Check sheet for the modelled part. Datum: model origin and axes. Units: mm. A direction names the side the tool comes from. Round coordinates to 2 decimals unless told otherwise and drop trailing zeros. Order: outer loops, then holes, each group sorted by start corner. A loop starts at its lowest first (then second) coordinate and runs counter-clockwise, first axis right, second up.
```python
from build123d import *

# Parameters (mm, degrees)
BOSS_EXTRUDE1_DEPTH         = 2
SKETCH5_R                   = 4
SKETCH5_R_2                 = 1.998542518
BOSS_EXTRUDE2_DEPTH         = 3
SKETCH8_R                   = 1.5
CUT_EXTRUDE2_DEPTH          = 30.027201103
CUT_EXTRUDE3_REACH          = 31.027
SKETCH10_R                  = 0.75
LPATTERN1_COUNT             = 4
LPATTERN1_PITCH             = 3.5
CIRPATTERN1_COUNT           = 4
CIRPATTERN1_COPY_1_REACH    = 31.027
CIRPATTERN1_COPY_1_SKETCH_R = 0.75
CIRPATTERN1_COPY_2_REACH    = 31.027
CIRPATTERN1_COPY_2_SKETCH_R = 0.75
CIRPATTERN1_COPY_3_REACH    = 31.027
CIRPATTERN1_COPY_3_SKETCH_R = 0.75
CIRPATTERN1_COPY_4_REACH    = 31.027
CIRPATTERN1_COPY_4_SKETCH_R = 0.75
CIRPATTERN1_COPY_5_REACH    = 31.027
CIRPATTERN1_COPY_5_SKETCH_R = 0.75
CIRPATTERN1_COPY_6_REACH    = 31.027
CIRPATTERN1_COPY_6_SKETCH_R = 0.75
CIRPATTERN1_COPY_7_REACH    = 31.027
CIRPATTERN1_COPY_7_SKETCH_R = 0.75
CIRPATTERN1_COPY_8_REACH    = 31.027
CIRPATTERN1_COPY_8_SKETCH_R = 0.75
CIRPATTERN1_COPY_9_REACH    = 31.027
CIRPATTERN1_COPY_9_SKETCH_R = 0.75


with BuildPart() as part:
    # Sketch1 → Boss-Extrude1 (new body)
    with BuildSketch(Plane(origin=(0, 0, 0), x_dir=(1, 0, 0), z_dir=(0, 1, 0))):
        with BuildLine():
            Line((11.195476756, 1.969359322), (4.786657556, -6.592741724))
            ThreePointArc((4.786657556, -6.592741724), (3.929987754, -8.118293207), (4.786657556, -9.643844691))
            Line((4.786657556, -9.643844691), (11.195476756, -18.205945736))
            ThreePointArc((11.195476756, -18.205945736), (10.933214648, -21.871520101), (7.267640283, -22.133782209))
            Line((7.267640283, -22.133782209), (-1.294460762, -15.724963009))
            ThreePointArc((-1.294460762, -15.724963009), (-2.820012246, -14.868293207), (-4.34556373, -15.724963009))
            Line((-4.34556373, -15.724963009), (-12.907664775, -22.133782209))
            ThreePointArc((-12.907664775, -22.133782209), (-16.57323914, -21.871520101), (-16.835501248, -18.205945736))
            Line((-16.835501248, -18.205945736), (-10.426682048, -9.643844691))
            ThreePointArc((-10.426682048, -9.643844691), (-9.570012246, -8.118293207), (-10.426682048, -6.592741724))
            Line((-10.426682048, -6.592741724), (-16.835501248, 1.969359322))
            ThreePointArc((-16.835501248, 1.969359322), (-16.57323914, 5.634933687), (-12.907664775, 5.897195795))
            Line((-12.907664775, 5.897195795), (-4.34556373, -0.511623405))
            ThreePointArc((-4.34556373, -0.511623405), (-2.820012246, -1.368293207), (-1.294460762, -0.511623405))
            Line((-1.294460762, -0.511623405), (7.267640283, 5.897195795))
            ThreePointArc((7.267640283, 5.897195795), (10.933214648, 5.634933687), (11.195476756, 1.969359322))
        make_face()
    extrude(amount=BOSS_EXTRUDE1_DEPTH)

    # Sketch5 → Boss-Extrude2 (add)
    with BuildSketch(Plane(origin=(0, 2, 0), x_dir=(1, 0, 0), z_dir=(0, 1, 0))):
        with Locations(Location((-2.820012246, -8.118293207, 0), (0, 0, 90))):
            Circle(SKETCH5_R)
        with Locations(Location((-2.820012246, -8.118293207, 0), (0, 0, 270))):
            Circle(SKETCH5_R_2, mode=Mode.SUBTRACT)
    extrude(amount=BOSS_EXTRUDE2_DEPTH)

    # Sketch8 → Cut-Extrude2 (cut, through all)
    with BuildSketch(Plane.XZ):
        with Locations(Location((-2.820012246, 8.118293207, 0), (0, 0, 270))):
            Circle(SKETCH8_R)
    extrude(amount=-CUT_EXTRUDE2_DEPTH, mode=Mode.SUBTRACT)

    # Sketch10 → Cut-Extrude3 (cut, up to next)
    with BuildSketch(Plane.XZ, mode=Mode.PRIVATE) as cut_extrude3_sk1:
        with Locations(Location((9.519001086, -4.220720125, 0), (0, 0, 270))):
            Circle(SKETCH10_R)
    cut_extrude3_tool1 = extrude(cut_extrude3_sk1.sketch, amount=-CUT_EXTRUDE3_REACH, mode=Mode.PRIVATE) & part.part
    cut_extrude3 = cut_extrude3_tool1.solids().sort_by_distance((9.519001, 0, -4.22072))[0]
    add(cut_extrude3, mode=Mode.SUBTRACT)

    # LPattern1: Cut-Extrude3 ×4
    with Locations(*[Vector(-0.707106781186547, 0, 0.707106781186548) * (i * LPATTERN1_PITCH) for i in range(1, LPATTERN1_COUNT)]):
        add(cut_extrude3, mode=Mode.SUBTRACT)

    # CirPattern1: Cut-Extrude3 ×4 about axis
    cirpattern1_axis = Axis((-2.820012246, 0, 8.118293207), (0, 1, 0))
    for i in range(1, CIRPATTERN1_COUNT):
        add(cut_extrude3.rotate(cirpattern1_axis, i * 360 / CIRPATTERN1_COUNT), mode=Mode.SUBTRACT)

    # CirPattern1 copy 1 sketch → CirPattern1 copy 1 (cut, up to next)
    with BuildSketch(Plane(origin=(-8.463431719, 0, 7.773154695), x_dir=(0, 0, -1), z_dir=(0, -1, 0)), mode=Mode.PRIVATE) as cirpattern1_copy_1_sk1:
        with Locations(Location((9.519001086, -4.220720125, 0), (0, 0, 270))):
            Circle(CIRPATTERN1_COPY_1_SKETCH_R)
    cirpattern1_copy_1_tool1 = extrude(cirpattern1_copy_1_sk1.sketch, amount=-CIRPATTERN1_COPY_1_REACH, mode=Mode.PRIVATE) & part.part
    add(cirpattern1_copy_1_tool1.solids().sort_by_distance((-12.684151719, 0, -1.745846305))[0], mode=Mode.SUBTRACT)

    # CirPattern1 copy 2 sketch → CirPattern1 copy 2 (cut, up to next)
    with BuildSketch(Plane(origin=(-3.165150758, 0, 13.76171268), x_dir=(-1, 0, 0), z_dir=(0, -1, 0)), mode=Mode.PRIVATE) as cirpattern1_copy_2_sk1:
        with Locations(Location((9.519001086, -4.220720125, 0), (0, 0, 270))):
            Circle(CIRPATTERN1_COPY_2_SKETCH_R)
    cirpattern1_copy_2_tool1 = extrude(cirpattern1_copy_2_sk1.sketch, amount=-CIRPATTERN1_COPY_2_REACH, mode=Mode.PRIVATE) & part.part
    add(cirpattern1_copy_2_tool1.solids().sort_by_distance((-12.684151758, 0, 17.98243268))[0], mode=Mode.SUBTRACT)

    # CirPattern1 copy 3 sketch → CirPattern1 copy 3 (cut, up to next)
    with BuildSketch(Plane(origin=(2.823407227, 0, 8.463431719), x_dir=(0, 0, 1), z_dir=(0, -1, 0)), mode=Mode.PRIVATE) as cirpattern1_copy_3_sk1:
        with Locations(Location((9.519001086, -4.220720125, 0), (0, 0, 270))):
            Circle(CIRPATTERN1_COPY_3_SKETCH_R)
    cirpattern1_copy_3_tool1 = extrude(cirpattern1_copy_3_sk1.sketch, amount=-CIRPATTERN1_COPY_3_REACH, mode=Mode.PRIVATE) & part.part
    add(cirpattern1_copy_3_tool1.solids().sort_by_distance((7.044127227, 0, 17.982432719))[0], mode=Mode.SUBTRACT)

    # CirPattern1 copy 4 sketch → CirPattern1 copy 4 (cut, up to next)
    with BuildSketch(Plane(origin=(-5.988557985, 0, 10.248028429), x_dir=(0, 0, -1), z_dir=(0, -1, 0)), mode=Mode.PRIVATE) as cirpattern1_copy_4_sk1:
        with Locations(Location((9.519001086, -4.220720125, 0), (0, 0, 270))):
            Circle(CIRPATTERN1_COPY_4_SKETCH_R)
    cirpattern1_copy_4_tool1 = extrude(cirpattern1_copy_4_sk1.sketch, amount=-CIRPATTERN1_COPY_4_REACH, mode=Mode.PRIVATE) & part.part
    add(cirpattern1_copy_4_tool1.solids().sort_by_distance((-10.209277985, 0, 0.729027429))[0], mode=Mode.SUBTRACT)

    # CirPattern1 copy 5 sketch → CirPattern1 copy 5 (cut, up to next)
    with BuildSketch(Plane(origin=(-0.690277024, 0, 11.286838946), x_dir=(-1, 0, 0), z_dir=(0, -1, 0)), mode=Mode.PRIVATE) as cirpattern1_copy_5_sk1:
        with Locations(Location((9.519001086, -4.220720125, 0), (0, 0, 270))):
            Circle(CIRPATTERN1_COPY_5_SKETCH_R)
    cirpattern1_copy_5_tool1 = extrude(cirpattern1_copy_5_sk1.sketch, amount=-CIRPATTERN1_COPY_5_REACH, mode=Mode.PRIVATE) & part.part
    add(cirpattern1_copy_5_tool1.solids().sort_by_distance((-10.209278024, 0, 15.507558946))[0], mode=Mode.SUBTRACT)

    # CirPattern1 copy 6 sketch → CirPattern1 copy 6 (cut, up to next)
    with BuildSketch(Plane(origin=(0.348533493, 0, 5.988557985), x_dir=(0, 0, 1), z_dir=(0, -1, 0)), mode=Mode.PRIVATE) as cirpattern1_copy_6_sk1:
        with Locations(Location((9.519001086, -4.220720125, 0), (0, 0, 270))):
            Circle(CIRPATTERN1_COPY_6_SKETCH_R)
    cirpattern1_copy_6_tool1 = extrude(cirpattern1_copy_6_sk1.sketch, amount=-CIRPATTERN1_COPY_6_REACH, mode=Mode.PRIVATE) & part.part
    add(cirpattern1_copy_6_tool1.solids().sort_by_distance((4.569253493, 0, 15.507558985))[0], mode=Mode.SUBTRACT)

    # CirPattern1 copy 7 sketch → CirPattern1 copy 7 (cut, up to next)
    with BuildSketch(Plane(origin=(-3.513684251, 0, 12.722902164), x_dir=(0, 0, -1), z_dir=(0, -1, 0)), mode=Mode.PRIVATE) as cirpattern1_copy_7_sk1:
        with Locations(Location((9.519001086, -4.220720125, 0), (0, 0, 270))):
            Circle(CIRPATTERN1_COPY_7_SKETCH_R)
    cirpattern1_copy_7_tool1 = extrude(cirpattern1_copy_7_sk1.sketch, amount=-CIRPATTERN1_COPY_7_REACH, mode=Mode.PRIVATE) & part.part
    add(cirpattern1_copy_7_tool1.solids().sort_by_distance((-7.734404251, 0, 3.203901164))[0], mode=Mode.SUBTRACT)

    # CirPattern1 copy 8 sketch → CirPattern1 copy 8 (cut, up to next)
    with BuildSketch(Plane(origin=(1.78459671, 0, 8.811965212), x_dir=(-1, 0, 0), z_dir=(0, -1, 0)), mode=Mode.PRIVATE) as cirpattern1_copy_8_sk1:
        with Locations(Location((9.519001086, -4.220720125, 0), (0, 0, 270))):
            Circle(CIRPATTERN1_COPY_8_SKETCH_R)
    cirpattern1_copy_8_tool1 = extrude(cirpattern1_copy_8_sk1.sketch, amount=-CIRPATTERN1_COPY_8_REACH, mode=Mode.PRIVATE) & part.part
    add(cirpattern1_copy_8_tool1.solids().sort_by_distance((-7.73440429, 0, 13.032685212))[0], mode=Mode.SUBTRACT)

    # CirPattern1 copy 9 sketch → CirPattern1 copy 9 (cut, up to next)
    with BuildSketch(Plane(origin=(-2.126340241, 0, 3.513684251), x_dir=(0, 0, 1), z_dir=(0, -1, 0)), mode=Mode.PRIVATE) as cirpattern1_copy_9_sk1:
        with Locations(Location((9.519001086, -4.220720125, 0), (0, 0, 270))):
            Circle(CIRPATTERN1_COPY_9_SKETCH_R)
    cirpattern1_copy_9_tool1 = extrude(cirpattern1_copy_9_sk1.sketch, amount=-CIRPATTERN1_COPY_9_REACH, mode=Mode.PRIVATE) & part.part
    add(cirpattern1_copy_9_tool1.solids().sort_by_distance((2.094379759, 0, 13.032685251))[0], mode=Mode.SUBTRACT)


solid = part.part
```
Item 1: Access from +Z, -Z, +X, -X, +Y, -Y to the whole of each face (thin tool, end or side, straight path). Record for faces 1 (the flat face through (8, 1, 2.3)), 2 (the flat face through (1, 2, 5)), 3 (the flat face through (-13.586, 0.986, 2.372)).
Answer:
face 1: +X, +Y, -Y
face 2: +Y
face 3: -X, +Y, -Y
Item 2: Sectioned sample at A-A (y = 0.9). State how many separate pieces and enclosed holes the cut face has, and give its area (3 significant figures).
Answer:
separate pieces: 1
enclosed holes: 17
area: 455 mm2
Item 3: Sectioned sample at C-C (y = 3.05). Record the cut outline in (x, z), and give its area (3 significant figures).
Answer:
outline: circle Ø8 at (-2.82, 8.12); hole circle Ø4 at (-2.82, 8.12)
area: 37.7 mm2
Item 4: Sectioned sample at B-B (x = -3.25). Record the cut outline in (y, z), and give its area (3 significant figures).
Answer:
outline: (0, 1.32) - (2, 1.32) - (2, 4.14) - (5, 4.14) - (5, 6.17) - (2, 6.17) - (2, 6.68) - (0, 6.68) - close; (0, 9.56) - (2, 9.56) - (2, 10.07) - (5, 10.07) - (5, 12.1) - (2, 12.1) - (2, 14.92) - (0, 14.92) - close
area: 33.6 mm2
Item 5: Sectioned sample at D-D (x = 0.25). Record the cut outline in (y, z), and give its area (3 significant figures).
Answer:
outline: (0, -0.64) - (2, -0.64) - (2, 5.55) - (5, 5.55) - (5, 10.68) - (2, 10.68) - (2, 16.88) - (0, 16.88) - close
area: 50.4 mm2
Item 6: Go/stop test with flat-tipped pins: P1, Ø2.5, axis at x = -15.16, z = -4.22, coming from the +Y side; P2, Ø2, axis at x = -3.5, z = 9, coming from the +Y side; P3, Ø2, axis at x = 7.5, z = 10, coming from the -Y side; P4, Ø1.5, axis at y = 1.5, z = 3.5, coming from the -X side. Record where each tip stops, or that it passes through.
Answer:
P1: stops at y = 2
P2: stops at y = 5
P3: passes through
P4: stops at x = -13.3
Item 7: Scan lines: line 1 along Z through (x, y) = (1.5, 1.05); line 2 along X through (y, z) = (1.2, 3.5); line 3 along Z through (x, y) = (-7.25, 1.4). Record each from-to range of solid material in increasing order.
Answer:
line 1: z = -1.58 to 2.75, 3.66 to 12.58, 13.49 to 17.82
line 2: x = -12.74 to -8.42, -7.05 to 1.41, 2.78 to 7.1
line 3: z = -1.66 to 2.63, 3.78 to 12.46, 13.61 to 17.9
Item 8: Release check for a two-part mould opening along Z. For faces 4 (the cylindrical face through (-2.79, 0.99, 14.87)), 5 (the cylindrical face through (11, 1, 21.8)), 6 (the flat face through (-3, 0, 5)), 7 (the cylindrical face through (-6.985, 0.986, 3.171)) record: released by +Z, released by -Z, zero draft, split by the parting line, or undercut.
Answer:
face 4: released by +Z
face 5: undercut
face 6: zero draft
face 7: undercut
